Job drawing, mm, ordinate dimensions from the low corner. One solid piece. Give positions to 0.01 mm unless a question says otherwise; leave off trailing zeros. Loops run counter-clockwise (first coordinate to the right, second up) from the corner with the lowest first, then second, coordinate; pieces in that order, holes last. Notation, with made-up numbers: M 77.5,23 L 112.5,23 A32 ccw 112.5,50 Z; hole C -34,-6 d7. An arc over 180 degrees is marked long. Answer in a Markdown table with one row per item.
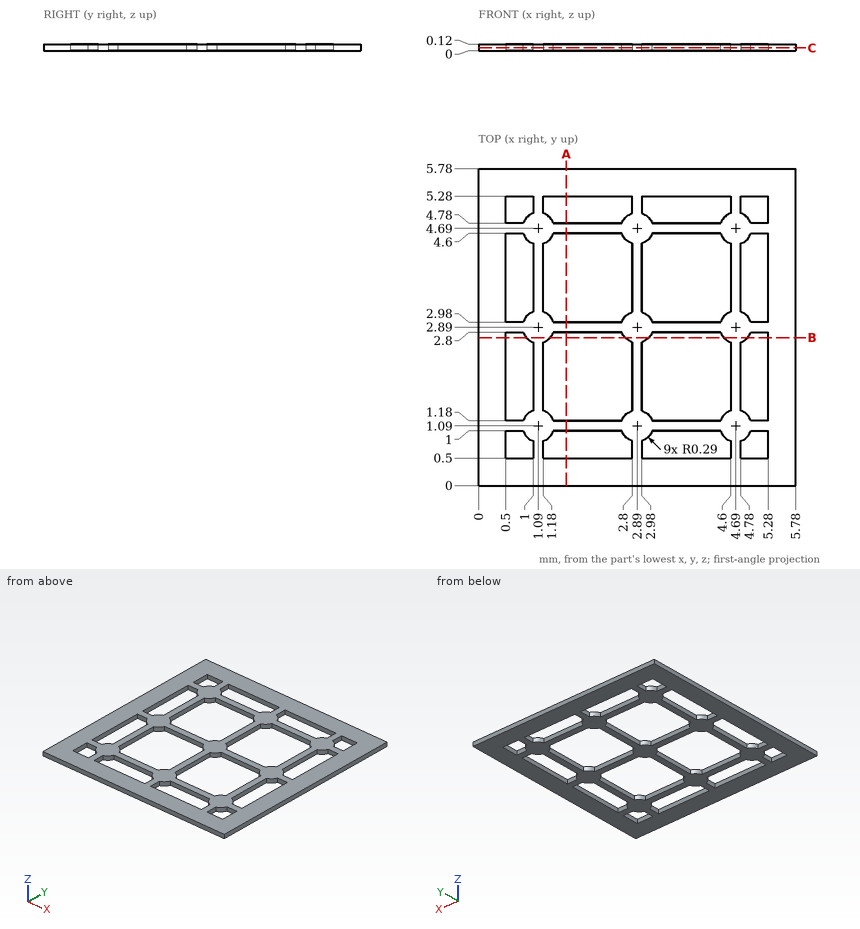
(1) Saw through at A-A (x = 1.6). Write the cut outline in (y, z).
Recorded:
| item | result |
|---|---|
| outline | M 0,0 L 0.5,0 L 0.5,0.12 L 0,0.12 Z; M 1,0 L 1.18,0 L 1.18,0.12 L 1,0.12 Z; M 2.8,0 L 2.98,0 L 2.98,0.12 L 2.8,0.12 Z; M 4.6,0 L 4.78,0 L 4.78,0.12 L 4.6,0.12 Z; M 5.28,0 L 5.78,0 L 5.78,0.12 L 5.28,0.12 Z |
(2) Saw through at C-C (z = 0.05). Give the number of separate pieces and of enclosed holes in the cut face, plus the area to 3 significant figures.
Recorded:
| item | result |
|---|---|
| separate pieces | 1 |
| enclosed holes | 16 |
| area | 16.3 mm^2 |
(3) Saw through at B-B (y = 2.7). Write the cut outline in (x, z).
Recorded:
| item | result |
|---|---|
| outline | M 0,0 L 0.5,0 L 0.5,0.12 L 0,0.12 Z; M 0.87,0 L 1.31,0 L 1.31,0.12 L 0.87,0.12 Z; M 2.67,0 L 3.11,0 L 3.11,0.12 L 2.67,0.12 Z; M 4.47,0 L 4.91,0 L 4.91,0.12 L 4.47,0.12 Z; M 5.28,0 L 5.78,0 L 5.78,0.12 L 5.28,0.12 Z |
(4) Drill centre line: line 1 along Y through (x, z) = (3.35, 0.05). Where is it in solid material? Low to high.
Recorded:
| item | result |
|---|---|
| line 1 | y = 0 to 0.5, 1 to 1.18, 2.8 to 2.98, 4.6 to 4.78, 5.28 to 5.78 |
